Part model, mm, in its own coordinate system. A direction names the side the tool comes from. Give positions to 0.01 mm unless a question says otherwise; leave off trailing zeros. Write each loop counter-clockwise with the first axis right and the second up, starting at its lowest first coordinate (ties: lowest second). Pieces come first, ordered by that corner, then holes. Notation, with made-up numbers: M 48,52 L 92,52 A23 ccw 92,71 Z; hole C 9,-21.75 d7. An arc over 180 degrees is marked long. Answer as CSV lines item,"result". Start each with the question number.
1) Mould opens along Y. For faces 4 (the flat face through (60, 25, 1)), 5 (the flat face through (1, -2, 1)), 6 (the flat face through (15, 27, 1)), 7 (the flat face through (-44, -13, 1)) say: pulls with the +Y half, pulls with the -Y half, needs draft (parallel to the pull), parting line crosses it, or undercut.
2) Slice it at A-A, the plane x = 30.5. Give the cut face in (y, z).
3) Pin check, flat tips, straight feed: pin 1 Ø12 at (x, y) = (6, -3) entering from -Z; pin 2 Ø0.9 at (y, z) = (-12, 1) entering from -X; pin 3 Ø0.9 at (y, z) = (-8.5, 1) entering from +X. Stop position of each tip, or through.
4) Slice it at B-B, the plane z = 1.6. Give the number of separate pieces and of enclosed holes in the cut face, plus the area to 3 significant figures.
5) Tool access for faces 1 (the flat face through (-20, -25, 1)), 2 (the flat face through (-59, -2, 1)), 3 (the flat face through (-40, 25, 1)): list every direction of +Z, -Z, +X, -X, +Y, -Y with a clear straight run to the whole face (end or side of a thin tool).
6) Wall check: line 1 along Y through (x, z) = (-18.5, 0.4); line 2 along Y through (x, z) = (-26.5, 0.9); line 3 along X through (y, z) = (9.5, 0.25). Give the ranges that are in metal, low to high. Write a range as from..to.
```python
from build123d import *

# Parameters (mm, degrees)
BOSS_EXTRUDE1_DEPTH = 3
SKETCH4_W           = 10
SKETCH4_H           = 11
CUT_EXTRUDE2_DEPTH  = 3


with BuildPart() as part:
    # Sketch1 → Boss-Extrude1 (new body)
    with BuildSketch(Plane.XY):
        Polygon((15, 28), (15, 25), (25, 25), (25, 28), (35, 28), (35, 25), (45, 25), (45, 28), (55, 28), (55, 25), (65, 25), (65, 28), (78, 28), (78, 15), (75, 15), (75, 5), (78, 5), (78, -5), (75, -5), (75, -15), (78, -15), (78, -28), (65, -28), (65, -25), (55, -25), (55, -28), (45, -28), (45, -25), (35, -25), (35, -28), (25, -28), (25, -25), (15, -25), (15, -28), (5, -28), (5, -25), (-5, -25), (-5, -28), (-15, -28), (-15, -25), (-25, -25), (-25, -28), (-35, -28), (-35, -25), (-45, -25), (-45, -28), (-55, -28), (-55, -25), (-65, -25), (-65, -28), (-78, -28), (-78, -15), (-75, -15), (-75, -5), (-78, -5), (-78, 5), (-75, 5), (-75, 15), (-78, 15), (-78, 28), (-65, 28), (-65, 25), (-55, 25), (-55, 28), (-45, 28), (-45, 25), (-35, 25), (-35, 28), (-25, 28), (-25, 25), (-15, 25), (-15, 28), (-5, 28), (-5, 25), (5, 25), (5, 28), align=None)
    extrude(amount=BOSS_EXTRUDE1_DEPTH)

    # Sketch4 → Cut-Extrude2 (cut)
    with BuildSketch(Plane(origin=(0, 0, 0), x_dir=(-1, 0, 0), z_dir=(0, 0, -1))):
        with Locations((-61, -7.5)):
            Rectangle(SKETCH4_W, SKETCH4_H)
        with Locations((-46, -7.5)):
            Rectangle(SKETCH4_W, SKETCH4_H)
        with Locations((-31, -7.5)):
            Rectangle(SKETCH4_W, SKETCH4_H)
        with Locations((-16, -7.5)):
            Rectangle(SKETCH4_W, SKETCH4_H)
        with Locations((-1, -7.5)):
            Rectangle(SKETCH4_W, SKETCH4_H)
        with Locations((14, -7.5)):
            Rectangle(SKETCH4_W, SKETCH4_H)
        with Locations((29, -7.5)):
            Rectangle(SKETCH4_W, SKETCH4_H)
        with Locations((44, -7.5)):
            Rectangle(SKETCH4_W, SKETCH4_H)
        with Locations((59, -7.5)):
            Rectangle(SKETCH4_W, SKETCH4_H)
    extrude(amount=-CUT_EXTRUDE2_DEPTH, mode=Mode.SUBTRACT)


solid = part.part
```
Found:
1,face 4,"pulls with the +Y half"
1,face 5,"undercut"
1,face 6,"needs draft"
1,face 7,"undercut"
2,outline,"M -28,0 L -13,0 L -13,3 L -28,3 Z; M -2,0 L 28,0 L 28,3 L -2,3 Z"
3,pin 1,"z = 0"
3,pin 2,"x = -75"
3,pin 3,"x = 75"
4,separate pieces,"1"
4,enclosed holes,"9"
4,area,"7,210 mm²"
5,face 1,"+Z, -Z, -Y"
5,face 2,"+Z, -Z"
5,face 3,"+Z, -Z, +Y"
6,line 1,"-25..-13, -2..25"
6,line 2,"-28..-13, -2..28"
6,line 3,"-75..75"
